Could you check a few things on this model? Use its own coordinates, in mm. Face numbers are marked on the shaded views. A direction names the side the tool comes from. Give positions to 0.01 mm unless a question says otherwise; leave off trailing zeros. Order: outer loops, then holes, each group sorted by start corner. A loop starts at its lowest first (then second) coordinate and runs counter-clockwise, first axis right, second up. Notation, with made-up numbers: M 77.5,82.25 L 121.5,82.25 A15 cw 121.5,103.25 Z; hole C 20,-25.75 d11. An arc over 180 degrees is marked long. Use a Markdown table: item, result. Add a question column.
Item 1: Suppose I cut it at A-A on x = 10. Write out the boundary of the cut face in (y, z).
Item 2: If I drill on L1, parallel to Y at x = 10, z = 2.1; L2, parallel to Y at x = 11.25, z = 1.2; L3, parallel to X at y = 14.5, z = 1.7, over which ranges is the centre line in solid material (lowest first)? Write a range as from..to.
Item 3: Suppose I cut it at B-B on y = 7. Write out the boundary of the cut face in (x, z).
Item 4: If we mould it in two halves opening along Y, with no side actions, what happens to the marked faces 3, 4, 5 and 6? For each: released by +Y, released by -Y, zero draft, split by the parting line, or undercut.
Item 5: For the marked faces 1 and 2, which set-ups out of +Z, -Z, +X, -X, +Y, -Y let a thin tool reach every point of the face, with its end or its side?
Item 6: I'm going to push flat-ended pins straight in: pin 1 Ø4 at (x, y) = (10, 7) entering from +Z; pin 2 Ø1.5 at (y, z) = (33.5, 3) entering from -X; pin 3 Ø1.5 at (y, z) = (26.5, 4) entering from +X. Where does each tip first touch, or does it pass through?
Item 7: Suppose I cut it at C-C on z = 2.85. Write out the boundary of the cut face in (x, y), plus the area to 3 significant figures.
Item 8: Suppose I cut it at D-D on y = 17. Write out the boundary of the cut face in (x, z), plus the area to 3 significant figures.
from build123d import *

# Parameters (mm, degrees)
SKETCH1_W            = 20
SKETCH1_H            = 50
BOSS_EXTRUDE1_DEPTH  = 5
SKETCH2_R            = 2.1
SKETCH2_R_2          = 1.1
CUT_EXTRUDE1_DEPTH   = 55.083269132
SKETCH3_W            = 3
SKETCH3_H            = 30
CUT_EXTRUDE2_DEPTH   = 55.083269132
FILLET1_R            = 5
FILLET1_OF_MIRROR1_R = 5
FILLET3_R            = 1


with BuildPart() as part:
    # Sketch1 → Boss-Extrude1 (new body)
    with BuildSketch(Plane.XY):
        with Locations((10, 25)):
            Rectangle(SKETCH1_W, SKETCH1_H)
    extrude(amount=BOSS_EXTRUDE1_DEPTH)

    # Sketch2 → Cut-Extrude1 (cut, through all)
    with BuildSketch(Plane.XY.offset(5)):
        with Locations((10, 43)):
            Circle(SKETCH2_R)
        with Locations((10, 7)):
            Circle(SKETCH2_R)
        with Locations((10, 29.75)):
            Circle(SKETCH2_R_2)
        with Locations((10, 20.25)):
            Circle(SKETCH2_R_2)
    extrude(amount=-CUT_EXTRUDE1_DEPTH, mode=Mode.SUBTRACT)

    # Sketch3 → Cut-Extrude2 (cut, through all)
    with BuildSketch(Plane.XY.offset(5)):
        with Locations((1.5, 25)):
            Rectangle(SKETCH3_W, SKETCH3_H)
    cut_extrude2 = extrude(amount=-CUT_EXTRUDE2_DEPTH, mode=Mode.SUBTRACT)

    # Fillet1
    # the kernel refuses this fillet: 5 mm, written as the material it adds along each edge
    with BuildSketch(Plane(origin=(3, 10, 5), x_dir=(-1, 0, 0), z_dir=(0, 0, -1))) as fillet1_piece_1:
        with BuildLine():
            CenterArc((5, 4.582575695), FILLET1_R, 180, 66.421821522)
            Line((0, 4.582575695), (-0.1, 4.582575695))
            Line((-0.1, 4.582575695), (-0.1, 0))
            Line((-0.1, 0), (0, -0.1))
            ThreePointArc((0, -0.1), (1.5, -0.1), (2.96, -0.091651514))
            Line((2.96, -0.091651514), (3, 0))
        make_face()
    extrude(amount=5)
    with BuildSketch(Plane(origin=(3, 40, 5), x_dir=(0, -1, 0), z_dir=(0, 0, -1))) as fillet1_piece_2:
        with BuildLine():
            CenterArc((4.582575695, 5), FILLET1_R, 203.578178478, 66.421821522)
            Line((0, 3), (-0.091651514, 2.96))
            ThreePointArc((-0.091651514, 2.96), (-0.1, 1.5), (-0.1, 0))
            Line((-0.1, 0), (0, -0.1))
            Line((0, -0.1), (4.582575695, -0.1))
            Line((4.582575695, -0.1), (4.582575695, 0))
        make_face()
    extrude(amount=5)

    # Mirror1: Cut-Extrude2 across plane
    add(cut_extrude2.mirror(Plane.ZY.offset(-10)), mode=Mode.SUBTRACT)

    # Fillet1 of Mirror1
    # the kernel refuses this fillet: 5 mm, written as the material it adds along each edge
    with BuildSketch(Plane(origin=(17, 10, 5), x_dir=(0, 1, 0), z_dir=(0, 0, -1))) as fillet1_of_mirror1_piece_1:
        with BuildLine():
            CenterArc((4.582575695, 5), FILLET1_OF_MIRROR1_R, 203.578178478, 66.421821522)
            Line((0, 3), (-0.091651514, 2.96))
            ThreePointArc((-0.091651514, 2.96), (-0.1, 1.5), (-0.1, 0))
            Line((-0.1, 0), (0, -0.1))
            Line((0, -0.1), (4.582575695, -0.1))
            Line((4.582575695, -0.1), (4.582575695, 0))
        make_face()
    extrude(amount=5)
    with BuildSketch(Plane(origin=(17, 40, 5), x_dir=(1, 0, 0), z_dir=(0, 0, -1))) as fillet1_of_mirror1_piece_2:
        with BuildLine():
            CenterArc((5, 4.582575695), FILLET1_OF_MIRROR1_R, 180, 66.421821522)
            Line((0, 4.582575695), (-0.1, 4.582575695))
            Line((-0.1, 4.582575695), (-0.1, 0))
            Line((-0.1, 0), (0, -0.1))
            ThreePointArc((0, -0.1), (1.5, -0.1), (2.96, -0.091651514))
            Line((2.96, -0.091651514), (3, 0))
        make_face()
    extrude(amount=5)

    # Fillet3
    fillet3_edges = [part.edges().sort_by_distance(p)[0] for p in [
        (20, 5, 5),
        (10, 50, 5),
        (0, 5, 0),
        (0, 5, 5),
        (0, 45, 5),
        (10, 50, 0),
        (3, 25, 5),
        (3, 25, 0),
        (20, 5, 0),
        (2.183300133, 11.843962907, 5),
        (2.183300133, 11.843962907, 0),
        (2.183300133, 38.156037093, 5),
        (2.183300133, 38.156037093, 0),
        (10, 0, 0),
        (0, 45, 0),
        (20, 45, 0),
        (20, 45, 5),
        (10, 0, 5),
        (17, 25, 5),
        (17, 25, 0),
        (17.816699867, 11.843962907, 5),
        (17.816699867, 11.843962907, 0),
        (17.816699867, 38.156037093, 5),
        (17.816699867, 38.156037093, 0),
    ]]
    fillet(fillet3_edges, radius=FILLET3_R)


solid = part.part
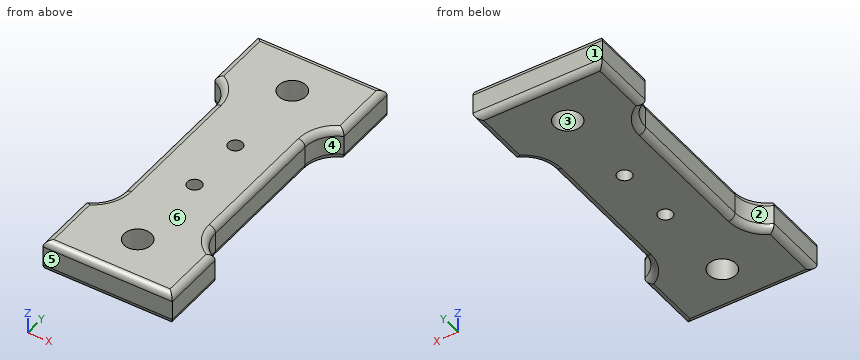
Findings below:
| question | item | result |
|---|---|---|
| 1 | outline | M 0,1 A1 ccw 1,0 L 4.9,0 L 4.9,5 L 1,5 A1 ccw 0,4 Z; M 9.1,0 L 19.15,0 L 19.15,5 L 9.1,5 Z; M 21.35,0 L 28.65,0 L 28.65,5 L 21.35,5 Z; M 30.85,0 L 40.9,0 L 40.9,5 L 30.85,5 Z; M 45.1,0 L 49,0 A1 ccw 50,1 L 50,4 A1 ccw 49,5 L 45.1,5 Z |
| 2 | L1 | y = 0..4.9, 9.1..19.15, 21.35..28.65, 30.85..40.9, 45.1..50 |
| 2 | L2 | y = 0..5.31, 8.69..41.31, 44.69..50 |
| 2 | L3 | x = 3..17 |
| 3 | outline | M 0,1 A1 ccw 1,0 L 7.9,0 L 7.9,5 L 1,5 A1 ccw 0,4 Z; M 12.1,0 L 19,0 A1 ccw 20,1 L 20,4 A1 ccw 19,5 L 12.1,5 Z |
| 4 | face 3 | undercut |
| 4 | face 4 | undercut |
| 4 | face 5 | released by -Y |
| 4 | face 6 | zero draft |
| 5 | face 1 | +Z, -Z, +X, -X, +Y |
| 5 | face 2 | +Z, -Z, -X |
| 6 | pin 1 | passes through |
| 6 | pin 2 | stops at x = 3 |
| 6 | pin 3 | stops at x = 17 |
| 7 | outline | M 0,0 L 20,0 L 20,10 A5 cw 17,14.58 L 17,35.42 A5 cw 20,40 L 20,50 L 0,50 L 0,40 A5 cw 3,35.42 L 3,14.58 A5 cw 0,10 Z; hole C 10,7 d4.2; hole C 10,43 d4.2; hole C 10,20.25 d2.2; hole C 10,29.75 d2.2 |
| 7 | area | 800 mm^2 |
| 8 | outline | M 3,1 A1 ccw 4,0 L 16,0 A1 ccw 17,1 L 17,4 A1 ccw 16,5 L 4,5 A1 ccw 3,4 Z |
| 8 | area | 69.1 mm^2 |
